from build123d import *

# Parameters (mm, degrees)
EXTRUDE_1_DEPTH     = 3
SKETCH_2_R          = 1.65
CUT_EXTRUDE_1_DEPTH = 3
FILLET_1_R          = 5
SKETCH_4_W          = 44.5
SKETCH_4_H          = 15.05
CUT_EXTRUDE_2_DEPTH = 0.5


with BuildPart() as part:
    # ｽｹｯﾁ1 → ﾎﾞｽ - 押し出し1 (new body)
    with BuildSketch(Plane.XY):
        Polygon((437.5, -0.909925586), (454.095389312, 5.13030215), (438.704482862, 47.416470085), (424.60909355, 42.286167935), (395, 0), (395, -16), (437.5, -16), align=None)
    extrude(amount=EXTRUDE_1_DEPTH)

    # ｽｹｯﾁ2 → ｶｯﾄ - 押し出し1 (cut)
    with BuildSketch(Plane.XY.offset(3)):
        with Locations((402.5, -8.5)):
            Circle(SKETCH_2_R)
        with Locations((432.5, -8.5)):
            Circle(SKETCH_2_R)
        with Locations((434.221939281, 37.803624354)):
            Circle(SKETCH_2_R)
        with Locations((444.482543581, 9.612845731)):
            Circle(SKETCH_2_R)
    extrude(amount=-CUT_EXTRUDE_1_DEPTH, mode=Mode.SUBTRACT)

    # ﾌｨﾚｯﾄ1
    fillet_1_edges = [part.edges().sort_by_distance(p)[0] for p in [
        (437.5, -16, 1.5),
        (395, -16, 1.5),
        (395, 0, 1.5),
        (424.60909355, 42.286167935, 1.5),
        (438.704482862, 47.416470085, 1.5),
        (454.095389312, 5.13030215, 1.5),
        (437.5, -0.909925586, 1.5),
    ]]
    fillet(fillet_1_edges, radius=FILLET_1_R)

    # ｽｹｯﾁ4 → ｶｯﾄ - 押し出し2 (cut)
    with BuildSketch(Plane.XY.offset(3)):
        Polygon((438.704482862, 47.416470085), (454.437409455, 4.190609529), (440.295035512, -0.956793628), (424.562108919, 42.269066928), align=None)
        with Locations((417.25, -8.475)):
            Rectangle(SKETCH_4_W, SKETCH_4_H)
    extrude(amount=-CUT_EXTRUDE_2_DEPTH, mode=Mode.SUBTRACT)


solid = part.part
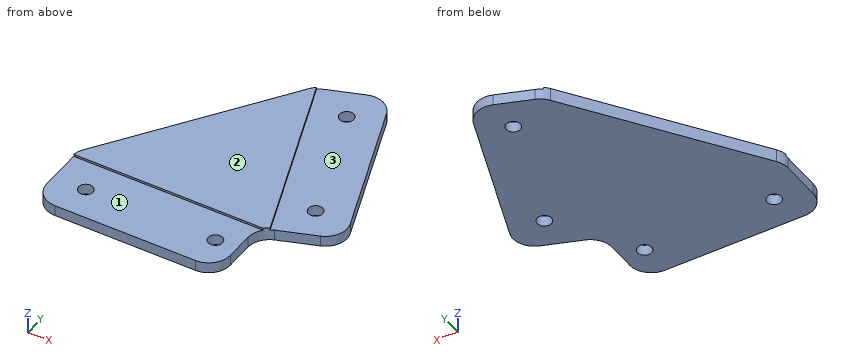
The listing builds one solid part. Answer for the finished solid, in the listing's coordinates (mm). Face numbers are marked on the shaded views. A direction names the side the tool comes from. Coordinates: 2 decimals unless noted, no trailing zeros. Loops run counter-clockwise (first coordinate to the right, second up) from the corner with the lowest first, then second, coordinate; pieces in that order, holes last. Notation, with made-up numbers: (-8, -12) -> (37, -12) arc R27 cw to (37, 6) -> close; hole circle Ø3 at (-22.75, 47.5). An arc over 180 degrees is marked (long way). Answer in a Markdown table with one row per item. Add a question column.
1. The part is cut by section B-B, the plane x = 408.5. Write down the section's boundary in (y, z).
2. The part is cut by section A-A, the plane y = -8.5. Write down the section's boundary in (x, z), then the cut area to 4 significant figures.
3. For the marked faces 1, 2 and 3, determine the directions among +Z, -Z, +X, -X, +Y, -Y from which every point of the face is accessible in a straight line to the end or side of a thin tool.
4. Flat-ended cylindrical pins translate along their axes: P1, Ø1.5, axis at x = 439, y = 18, coming from the -Z side; P2, Ø2, axis at x = 434.22, y = 37.8, coming from the +Z side; P3, Ø0.6, axis at x = 407.5, z = 3, coming from the -Y side; P4, Ø1.2, axis at y = -7.5, z = 2, coming from the +X side. Find the tip coordinate at first contact, or state that the pin passes through.
5. The part is cut by section C-C, the plane z = 1.3. Write down the section's boundary in (x, y), then the cut area to 3 significant figures.
6. Consider line 1 (Y direction, x = 433, z = 2.05); line 2 (Z direction, x = 404.5, y = -11); line 3 (Y direction, x = 425.5, z = 1.6). Determine where each line is inside the solid, lowest interval first. Write a range as [from, to].
7. The part is cut by section D-D, the plane y = 13. Write down the section's boundary in (x, z).
Answer below:
| question | item | result |
|---|---|---|
| 1 | outline | (-16, 0) -> (19.28, 0) -> (19.28, 3) -> (-0.95, 3) -> (-0.95, 2.5) -> (-16, 2.5) -> close |
| 2 | outline | (395, 0) -> (400.85, 0) -> (400.85, 2.5) -> (395, 2.5) -> close; (404.15, 0) -> (430.85, 0) -> (430.85, 2.5) -> (404.15, 2.5) -> close; (434.15, 0) -> (437.5, 0) -> (437.5, 2.5) -> (434.15, 2.5) -> close |
| 2 | area | 89.75 mm2 |
| 3 | face 1 | +Z, +X, -X, -Y |
| 3 | face 2 | +Z, +X, -X, +Y, -Y |
| 3 | face 3 | +Z, +X, +Y |
| 4 | P1 | z = 0 |
| 4 | P2 | through |
| 4 | P3 | y = -0.95 |
| 4 | P4 | x = 437.5 |
| 5 | outline | (395, -11) arc R5 ccw to (400, -16) -> (432.5, -16) arc R5 ccw to (437.5, -11) -> (437.5, -4.41) arc R5 cw to (440.79, 0.29) -> (449.4, 3.42) arc R5 ccw to (452.39, 9.83) -> (440.41, 42.72) arc R5 ccw to (434.01, 45.71) -> (426.09, 42.83) arc R5 ccw to (423.7, 40.99) -> (395.9, 1.29) arc R5 ccw to (395, -1.58) -> close; hole circle Ø3.3 at (402.5, -8.5); hole circle Ø3.3 at (432.5, -8.5); hole circle Ø3.3 at (434.22, 37.8); hole circle Ø3.3 at (444.48, 9.61) |
| 5 | area | 2,250 mm2 |
| 6 | line 1 | [-15.97, -10.07], [-6.93, 36.69], [38.91, 45.34] |
| 6 | line 2 | [0, 2.5] |
| 6 | line 3 | [-16, 42.57] |
| 7 | outline | (404.1, 0) -> (451.23, 0) -> (451.23, 2.5) -> (435.22, 2.5) -> (435.22, 3) -> (404.1, 3) -> close |
